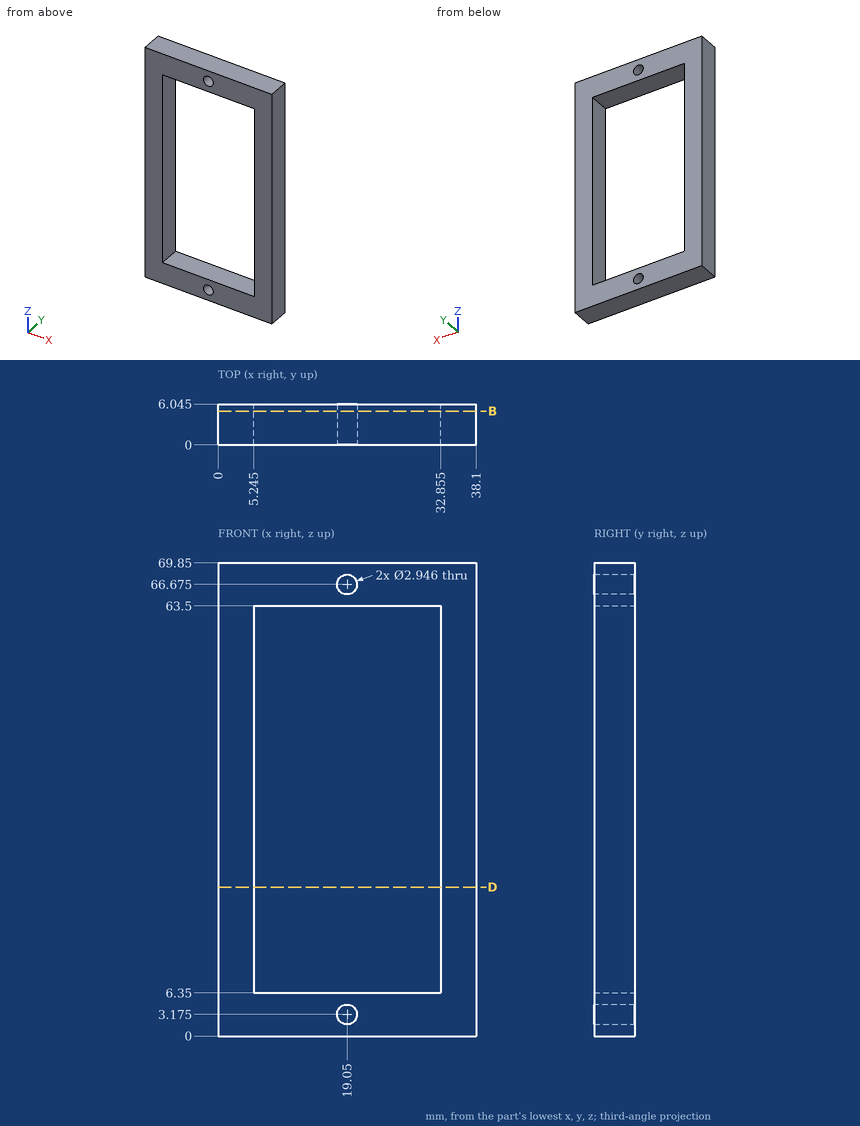
The drawing under review shows one solid part. Ordinate dimensions are in mm from its lowest x, y, z. Give positions to 0.01 mm unless a question says otherwise; leave off trailing zeros. Write each loop counter-clockwise with the first axis right and the second up, starting at its lowest first coordinate (ties: lowest second). Pieces come first, ordered by that corner, then holes. Notation, with made-up numbers: (70.5, 10.5) - (100.5, 10.5) arc R15 ccw to (100.5, 22.5) - close; hole circle Ø2 at (59.25, 14.5). An arc over 180 degrees is marked (long way). Answer in a Markdown table with one row per item. Add a question column.
1. We need section B-B on y = 5. State how many separate pieces and enclosed holes the cut face has, then the cut area to 3 significant figures.
2. We need section D-D on z = 22. Write out the cut boundary in (x, y) (1 decimal).
3. Insertion check: P1, Ø10, axis at x = 5.5, z = 35.5, coming from the +Y side (1 decimal). The pin has a flat end and moves straight along its axis. Give the tip position at first contact, or say it passes through.
4. Wall thickness on line 1 along X through (y, z) = (1.5, 25) (1 decimal); line 2 along Z through (x, y) = (25.5, 3); line 3 along Z through (x, y) = (19, 4.75): over which ranges is each line inside the solid? List them lowest first. Write a range as [from, to].
Ans:
| question | item | result |
|---|---|---|
| 1 | separate pieces | 1 |
| 1 | enclosed holes | 3 |
| 1 | area | 1,070 mm^2 |
| 2 | outline | (0, 0) - (5.2, 0) - (5.2, 6) - (0, 6) - close; (32.9, 0) - (38.1, 0) - (38.1, 6) - (32.9, 6) - close |
| 3 | P1 | stops at y = 6 |
| 4 | line 1 | x = [0, 5.2], [32.9, 38.1] |
| 4 | line 2 | z = [0, 6.35], [63.5, 69.85] |
| 4 | line 3 | z = [0, 1.7], [4.65, 6.35], [63.5, 65.2], [68.15, 69.85] |
